```python
from build123d import *

# Parameters (mm, degrees)
F1_DEPTH = 25


# Not quite as in the source:
# - a feature names something its author has since deleted; it is built from what else it names


with BuildPart() as f1:
    # F0 (on Front) → F1 (new body)
    with BuildSketch(Plane.XZ):
        with BuildLine():
            Line((-38.1111986935, 28.9119444788), (-38.1111986935, 0))
            Line((-38.1111986935, 0), (-27.9069803655, 0))
            Line((-27.9069803655, 0), (-27.9069803655, 28.9119444788))
            ThreePointArc((-27.9069803655, 28.9119444788), (-33.0090895295, 32.0041291416), (-38.1111986935, 28.9119444788))
        make_face()
        with BuildLine():
            Line((-0.1111986935, 28.9119444788), (-0.1111986935, 0))
            Line((-0.1111986935, 0), (10.0930196345, 0))
            Line((10.0930196345, 0), (10.0930196345, 28.9119444788))
            ThreePointArc((10.0930196345, 28.9119444788), (4.9909104705, 32.0041291416), (-0.1111986935, 28.9119444788))
        make_face()
        with BuildLine():
            Line((37.8888013065, 28.9119444788), (37.8888013065, 0))
            Line((37.8888013065, 0), (48.0930196345, 0))
            Line((48.0930196345, 0), (48.0930196345, 28.9119444788))
            ThreePointArc((48.0930196345, 28.9119444788), (42.9909104705, 32.0041291416), (37.8888013065, 28.9119444788))
        make_face()
        with BuildLine():
            Line((75.8888013065, 28.9119444788), (75.8888013065, 0))
            Line((75.8888013065, 0), (86.0930196345, 0))
            Line((86.0930196345, 0), (86.0930196345, 28.9119444788))
            ThreePointArc((86.0930196345, 28.9119444788), (80.9909104705, 32.0041291416), (75.8888013065, 28.9119444788))
        make_face()
        with BuildLine():
            Line((113.8888013065, 0), (124.0930196345, 0))
            Line((124.0930196345, 0), (124.0930196345, 28.9119444788))
            ThreePointArc((124.0930196345, 28.9119444788), (118.9909104705, 32.0041291416), (113.8888013065, 28.9119444788))
            Line((113.8888013065, 28.9119444788), (113.8888013065, 0))
        make_face()
        with BuildLine():
            Line((151.8888013065, 0), (162.0930196345, 0))
            Line((162.0930196345, 0), (162.0930196345, 28.9119444788))
            ThreePointArc((162.0930196345, 28.9119444788), (156.9909104705, 32.0041291416), (151.8888013065, 28.9119444788))
            Line((151.8888013065, 28.9119444788), (151.8888013065, 0))
        make_face()
        Polygon((-27.9069803655, 0), (-38.1111986935, 0), (-38.1111986935, -3.615781432), (162.0930196345, -3.615781432), (162.0930196345, 0), (151.8888013065, 0), (146.6320851445, 0), (131.5820539594, 0), (124.0930196345, 0), (113.8888013065, 0), (108.6320851445, 0), (93.5820539594, 0), (86.0930196345, 0), (75.8888013065, 0), (70.6320851445, 0), (55.5820539594, 0), (48.0930196345, 0), (37.8888013065, 0), (32.6320851445, 0), (10.0930196345, 0), (-0.1111986935, 0), (-5.3679148555, 0), align=None)
    extrude(amount=F1_DEPTH)


solid = f1.part
```
Design review of the part built by this model. Coordinates are the model's own, in mm. A direction names the side the tool comes from. Round coordinates to 2 decimals unless told otherwise and drop trailing zeros. Write each loop counter-clockwise with the first axis right and the second up, starting at its lowest first coordinate (ties: lowest second). Pieces come first, ordered by that corner, then holes.
Item 1: For probe 1 along X at (y, z) = (-11.5, 4); probe 2 along Z at (x, y) = (64, -1.75); probe 3 along Z at (x, y) = (118, -17.75), list the stretches that pass through material, from the lowest coordinate up.
Item 2: Clearance check with a flat-ended pin moving along its axis: pin 1 Ø12.5 at (x, y) = (139, -16.5) entering from +Z. State where the tip first meets the part, or that it passes through.
Item 3: We need section C-C on x = 92.5. Write out the cut boundary in (y, z), and give its area (3 significant figures).
Item 4: For faces 4 (the flat face through (75.889, -12, 15)), 5 (the flat face through (61, -12, -3.616)), list the 3-axis set-ups (+Z, -Z, +X, -X, +Y, -Y) from which the entire face can be reached by the end or side of a thin tool; tool diameter is ignored.
Item 5: The part is to be moulded in two halves that separate along X. For faces 1 (the flat face through (-38.111, -12, 13)), 2 (the flat face through (86.093, -12, 14)), 3 (the flat face through (38.3, 0, 10.5)), say which applies: +X half, -X half, draft (parallel to the pull), parting line (faces both ways), or undercut.
Item 6: We need section A-A on z = 2. Write out the cut boundary in (x, y), and give its area (3 significant figures).
Item 7: We need section B-B on y = -6.75. Write out the cut boundary in (x, z), and give its area (3 significant figures).
Returned:
1. probe 1: x = -38.11 to -27.91, -0.11 to 10.09, 37.89 to 48.09, 75.89 to 86.09, 113.89 to 124.09, 151.89 to 162.09
1. probe 2: z = -3.62 to 0
1. probe 3: z = -3.62 to 31.92
2. pin 1: stops at z = 0
3. outline: (-25, -3.62) - (0, -3.62) - (0, 0) - (-25, 0) - close
3. area: 90.4 mm2
4. face 4: +Z, +Y, -Y
4. face 5: -Z, +X, -X, +Y, -Y
5. face 1: -X half
5. face 2: undercut
5. face 3: draft
6. outline: (-38.11, -25) - (-27.91, -25) - (-27.91, 0) - (-38.11, 0) - close; (-0.11, -25) - (10.09, -25) - (10.09, 0) - (-0.11, 0) - close; (37.89, -25) - (48.09, -25) - (48.09, 0) - (37.89, 0) - close; (75.89, -25) - (86.09, -25) - (86.09, 0) - (75.89, 0) - close; (113.89, -25) - (124.09, -25) - (124.09, 0) - (113.89, 0) - close; (151.89, -25) - (162.09, -25) - (162.09, 0) - (151.89, 0) - close
6. area: 1,530 mm2
7. outline: (-38.11, -3.62) - (162.09, -3.62) - (162.09, 28.91) arc R5.76 ccw to (151.89, 28.91) - (151.89, 0) - (124.09, 0) - (124.09, 28.91) arc R5.76 ccw to (113.89, 28.91) - (113.89, 0) - (86.09, 0) - (86.09, 28.91) arc R5.76 ccw to (75.89, 28.91) - (75.89, 0) - (48.09, 0) - (48.09, 28.91) arc R5.76 ccw to (37.89, 28.91) - (37.89, 0) - (10.09, 0) - (10.09, 28.91) arc R5.76 ccw to (-0.11, 28.91) - (-0.11, 0) - (-27.91, 0) - (-27.91, 28.91) arc R5.76 ccw to (-38.11, 28.91) - close
7. area: 2,630 mm2
